from build123d import *

# Parameters (mm, degrees)
EXTRUDE099_DEPTH = 21
SKETCH081_W      = 143.5
SKETCH081_H      = 17.68
SKETCH081_W_2    = 32
SKETCH081_H_2    = 4
EXTRUDE073_DEPTH = 2


with BuildPart() as body060:
    # Sketch109 → Extrude099 (new body)
    with BuildSketch(Plane(origin=(178.5, 0, 0), x_dir=(0, -1, 0), z_dir=(-1, 0, 0))):
        Polygon((-212.5, 6.32), (-204, 6.32), (-204, 5.32), (-211.5, 5.32), (-211.5, -25), (-212.5, -25), align=None)
    extrude(amount=EXTRUDE099_DEPTH)


with BuildPart() as cut012:
    # Sketch081 → Extrude073 (new body)
    with BuildSketch(Plane.XZ.offset(-211.5)):
        with Locations((108.75, -16.16)):
            Rectangle(SKETCH081_W, SKETCH081_H)
        with Locations((131, -18.5)):
            Rectangle(SKETCH081_W_2, SKETCH081_H_2, mode=Mode.SUBTRACT)
    extrude(amount=-EXTRUDE073_DEPTH)

    # Cut012: cut Body060
    add(body060.part, mode=Mode.SUBTRACT)


solid = cut012.part
Geometry: final body of the model. Coordinates: model frame, mm. Coordinates: 2 decimals unless noted, no trailing zeros. Order: outer loops, then holes, each group sorted by start corner. A loop starts at its lowest first (then second) coordinate and runs counter-clockwise, first axis right, second up. Notation, with made-up numbers: (-14, 4) - (-9, 4) arc R30 cw to (-9, 42) - close; hole circle Ø4 at (63.25, -36). An arc over 180 degrees is marked (long way). Use one line per item in the form item = value.
1) Ray query, L1, parallel to X at y = 211.6, z = -17.5; L2, parallel to X at y = 211.9, z = -16.25; L3, parallel to X at y = 212.75, z = -19.5. Return the intervals inside material, ascending.
Solutions:
L1 = 37 to 115, 147 to 157.5, 178.5 to 180.5
L2 = 37 to 157.5, 178.5 to 180.5
L3 = 37 to 115, 147 to 180.5
2) Pin query (flat end, axial travel): pin 1 (5.5 mm diameter, centred on x = 172, z = -17, fed in from -Y). Return the tip coordinate at first contact, or that it passes through.
Solutions:
pin_1 = 212.5
3) Section A-A (y = 211.8). Return loops of the section in (x, z).
Solutions:
outline = (37, -25) - (157.5, -25) - (157.5, -7.32) - (37, -7.32) - close; (178.5, -25) - (180.5, -25) - (180.5, -7.32) - (178.5, -7.32) - close; hole (115, -20.5) - (147, -20.5) - (147, -16.5) - (115, -16.5) - close
4) Section C-C (x = 126.5). Return loops of the section in (y, z).
Solutions:
outline = (211.5, -25) - (213.5, -25) - (213.5, -20.5) - (211.5, -20.5) - close; (211.5, -16.5) - (213.5, -16.5) - (213.5, -7.32) - (211.5, -7.32) - close
5) Mould query, pull axis X, two halves, no side actions, for faces 1 (the face through (168, 212.5, -16)), 2 (the face through (108, 213.5, -16)). Classes: +X half, -X half, draft (parallel to the pull), parting line (faces both ways), or undercut.
Solutions:
face_1 = undercut
face_2 = draft
6) Section B-B (z = -18). Return loops of the section in (x, y), then the cut area to 3 significant figures.
Solutions:
outline = (37, 211.5) - (115, 211.5) - (115, 213.5) - (37, 213.5) - close; (147, 211.5) - (157.5, 211.5) - (157.5, 212.5) - (178.5, 212.5) - (178.5, 211.5) - (180.5, 211.5) - (180.5, 213.5) - (147, 213.5) - close
area = 202 mm^2
7) Section D-D (z = -23.5). Return loops of the section in (x, y).
Solutions:
outline = (37, 211.5) - (157.5, 211.5) - (157.5, 212.5) - (178.5, 212.5) - (178.5, 211.5) - (180.5, 211.5) - (180.5, 213.5) - (37, 213.5) - close
